from build123d import *

# Parameters (mm, degrees)
BASE_EXTRUDE_DEPTH    = 2.5
CORTE_EXTRUS_O1_DEPTH = 10


with BuildPart() as part:
    # Sketch1 → Base-Extrude (new, symmetric)
    with BuildSketch(Plane.XY):
        Polygon((-5.154154548, -4), (-7.6, 4), (0, 4), (0, 3.5), (23.165615911, 3.019042465), (25, -2.980957535), (0, -3.5), (0, -4), align=None)
    extrude(amount=BASE_EXTRUDE_DEPTH, both=True)

    # Esboço1 → Corte-extrusão1 (cut, along a direction that is not the sketch's normal)
    with BuildSketch(Plane(origin=(0, 4, 0), x_dir=(1, 0, 0), z_dir=(0, 1, 0))):
        Polygon((-5.94, -2.5), (-7.6, -0.84), (-7.6, -2.5), align=None)
        Polygon((-5.94, 2.5), (-7.6, 0.84), (-7.6, 2.5), align=None)
    extrude(amount=-CORTE_EXTRUS_O1_DEPTH, dir=(-0.29237170472273044, 0.9563047559630375, 0), mode=Mode.SUBTRACT)


solid = part.part
Read the model definition and answer for the solid it produces. Units are mm, in the model's axes. Round coordinates to 2 decimals unless told otherwise and drop trailing zeros. Write each loop counter-clockwise with the first axis right and the second up, starting at its lowest first coordinate (ties: lowest second). Pieces come first, ordered by that corner, then holes. Notation, with made-up numbers: M 83,63 L 108,63 A12 cw 108,79 Z; hole C 61.25,20 d10. An arc over 180 degrees is marked long. Use a Markdown table: item, result.
1) Flat-ended cylindrical pins translate along their axes: pin 1 (1.5 mm diameter, centred on y = 1.5, z = 0.5, fed in from +X); pin 2 (1 mm diameter, centred on x = 4, z = 0.5, fed in from -Y); pin 3 (1 mm diameter, centred on x = 2.5, z = -1.5, fed in from -Y). Find the tip coordinate at first contact, or state that the pin passes through.
Answers follow:
| item | result |
|---|---|
| pin 1 | stops at x = 23.86 |
| pin 2 | stops at y = -3.43 |
| pin 3 | stops at y = -3.46 |
2) For a pull along X with two mould halves and no side action, classify faces 1 (the flat face through (-6.36, -0.06, 0.01)), 2 (the flat face through (10, 0, 2.5)), 3 (the flat face through (24.07, 0.06, 0.04)) as pulls with the +X half, pulls with the -X half, needs draft (parallel to the pull), parting line crosses it, or undercut.
Answers follow:
| item | result |
|---|---|
| face 1 | pulls with the -X half |
| face 2 | needs draft |
| face 3 | pulls with the +X half |
3) The part is cut by section D-D (z = -1.85). Write down the section's boundary in (x, y), plus the area to 3 significant figures.
Answers follow:
| item | result |
|---|---|
| outline | M -6.59,4 L -4.14,-4 L 0,-4 L 0,-3.5 L 25,-2.98 L 23.17,3.02 L 0,3.5 L 0,4 Z |
| area | 199 mm2 |
4) The part is cut by section A-A (z = -0.15). Write down the section's boundary in (x, y).
Answers follow:
| item | result |
|---|---|
| outline | M -7.6,4 L -5.15,-4 L 0,-4 L 0,-3.5 L 25,-2.98 L 23.17,3.02 L 0,3.5 L 0,4 Z |
5) The part is cut by section B-B (y = 2.5). Write down the section's boundary in (x, z).
Answers follow:
| item | result |
|---|---|
| outline | M -7.14,-0.84 L -5.48,-2.5 L 23.32,-2.5 L 23.32,2.5 L -5.48,2.5 L -7.14,0.84 Z |
6) The part is cut by section C-C (x = 3.5). Write down the section's boundary in (y, z).
Answers follow:
| item | result |
|---|---|
| outline | M -3.43,-2.5 L 3.43,-2.5 L 3.43,2.5 L -3.43,2.5 Z |
7) Straight lines are drawn through the part: line 1 along Y through (x, z) = (6.5, -0.75); line 2 along X through (y, z) = (2.5, 1.1); line 3 along Y through (x, z) = (17, -1.1). For each, find the intervals that lie inside material, in ascending order. Write a range as [from, to].
Answers follow:
| item | result |
|---|---|
| line 1 | y = [-3.37, 3.37] |
| line 2 | x = [-6.88, 23.32] |
| line 3 | y = [-3.15, 3.15] |
